For this review, take the finished solid that the model builds, in its own axes (mm). A direction names the side the tool comes from. Give positions to 0.01 mm unless a question says otherwise; leave off trailing zeros. Loops run counter-clockwise (first coordinate to the right, second up) from the corner with the lowest first, then second, coordinate; pieces in that order, holes last. Notation, with made-up numbers: M 11.5,60 L 16.5,60 A20 cw 16.5,99 Z; hole C 20.25,9 d2. An arc over 180 degrees is marked long. Use CSV: the item, a comma, the result in double quotes. Start each with the question number.
1. To check wall thickness, follow line 1 (X direction, y = -16, z = 1.65); line 2 (X direction, y = 78, z = -4); line 3 (Z direction, x = -7, y = -17). State the ranges of each line that lie inside material, in increasing order. Write a range as [from, to].
2. Take a section at A-A, the plane y = 31.5. Write out the cut boundary in (x, z), and give its area (3 significant figures).
3. Insertion check: P1, Ø12, axis at y = 23.5, z = -4.5, coming from the +X side; P2, Ø1.7, axis at x = 3.85, y = -22.66, coming from the -Z side; P3, Ø8, axis at x = -1, y = -6, coming from the +Z side. Each pin has a flat end and moves straight along its axis. Give the tip position at first contact, or say it passes through.
4. Take a section at B-B, the plane z = 25.5. Write out the cut boundary in (x, y), and give its area (3 significant figures).
5. Tool access review of faces 1 (the face through (-17, 66, 2)), 2 (the face through (-2, 0, 2)), 3 (the face through (-7, -5, 3)), 4 (the face through (-15, 50, -20)), 5 (the face through (-16, 100, 2)): name each direction out of +Z, -Z, +X, -X, +Y, -Y from which nothing blocks a thin tool from reaching the whole face with its end or side.
Autodesk Inventor part; units mm, degrees
ref_plane "YZ Plane" through (0, 0, 0) normal (1, 0, 0) x (0, 1, 0)
ref_plane "XZ Plane" through (0, 0, 0) normal (0, 1, 0) x (-1, 0, 0)
ref_plane "XY Plane" through (0, 0, 0) normal (0, 0, 1) x (1, 0, 0)
sketch "Sketch1" plane through (0, 0, 0) normal (0, 0, 1) x (1, 0, 0)
  line L0 (-9, 25) -> (9, 25)
  line L1 (9, 25) -> (9, -25)
  line L2 (9, -25) -> (-9, -25)
  line L3 (-9, -25) -> (-9, 25)
  point P0 (0, 0)
  point P1 (0, 25)
  point P2 (-9, 0)
  dimension "d0" = 18
  dimension "d1" = 50
extrude "Extrusion1" add sketch "Sketch1" along normal blind 3
sketch "Sketch2" plane through (0, 0, 3) normal (0, 0, 1) x (1, 0, 0)
  circle A0 centre (0, -16) radius 9
  circle A1 centre (0, 16) radius 9
  line L0 (-9, -25) -> (9, -25)
  circle A2 centre (0, -8.304) radius 0.75
  line L1 (9, 25) -> (-9, 25)
  point P0 (0, 0)
  point P1 (-4, -25)
  point P2 (4, -25)
  point P3 (4, 25)
  point P4 (-4, 25)
  dimension "d6" = 18
  dimension "d8" = 1.5
  dimension "d10" = 18
extrude "Extrusion2" cut sketch "Sketch2" against normal up to surface (3 mm away) contours A2
pattern_circular "Circular Pattern1" count 12 over 360 about axis through (0, -16, 3) along (0, 0, 1) of "Extrusion2"
sketch "Sketch7" plane through (0, 0, 3) normal (0, 0, 1) x (1, 0, 0)
  line L0 (-19, 0) -> (11, 0)
  line L1 (11, 0) -> (11, 28.3489)
  line L2 (11, 28.3489) -> (-19, 28.3489)
  line L3 (-19, 28.3489) -> (-19, 0)
  line L4 (-9, -25) -> (9, -25)
  line L5 (-9, 25) -> (-9, -25)
  line L6 (9, -25) -> (9, 25)
  point P0 (0, 0)
  point P1 (-4, -25)
  point P2 (4, -25)
  point P3 (-9, 20)
  point P4 (-9, -20)
  point P5 (9, -20)
  dimension "d44" = 25
  dimension "d48" = 30
  dimension "d49" = 2
extrude "Extrusion8" cut sketch "Sketch7" against normal up to surface (3 mm away) contours L3 L2 L1 L0
ref_plane "Work Plane1" through (-9, -20, 0) normal (-1, 0, 0) x (0, 0, 1)
sketch "Sketch9" plane through (-9, -20, 0) normal (-1, 0, 0) x (0, 0, 1)
  line L0 (3, 0) -> (3, 20)
  line L1 (3, 20) -> (0, 20)
  line L2 (0, 20) -> (0, 0)
  line L3 (3, 0) -> (3, -5)
  line L4 (3, -5) -> (0, -5)
  line L5 (0, -5) -> (3, -5)
  line L6 (0, -5) -> (0, 0)
extrude "Extrusion9" add sketch "Sketch9" along normal blind 8
fillet "Fillet3" radius 5 1 edges at (9, -25, 1.5)
sketch "Sketch10" plane through (9, 0, 3) normal (0, 1, 0) x (1, 0, 0)
  line L0 (-5, 3) -> (-26, 3)
  line L1 (-26, 0) -> (-23, 0)
  line L2 (-23, 0) -> (-23, 3)
  line L3 (-23, 3) -> (-26, 3)
  line L4 (-26, 3) -> (-26, 0)
  point P0 (-9, 3)
  dimension "d53" = 3
extrude "Extrusion10" add sketch "Sketch10" along normal blind 70
fillet "Fillet4" radius 5 1 edges at (-17, -25, 1.5)
sketch "Sketch11" plane through (0, 0, 3) normal (0, 0, 1) x (1, 0, 0)
  line L0 (-14, 0) -> (-14, 70)
  line L1 (-17, 70) -> (-14, 70)
  line L2 (-14, 70) -> (-14, 50)
  line L3 (-14, 50) -> (-17, 50)
  line L4 (-17, 50) -> (-17, 70)
  point P0 (0, 0)
  dimension "d57" = 20
extrude "Extrusion11" add sketch "Sketch11" along normal blind 30
sketch "Sketch12" plane through (0, 0, 0) normal (0, 0, -1) x (-1, 0, 0)
  line L0 (14, 0) -> (14, 70)
  line L1 (17, 70) -> (14, 70)
  line L2 (14, 70) -> (14, 50)
  line L3 (14, 50) -> (17, 50)
  line L4 (17, 50) -> (17, 70)
  point P0 (0, 0)
  dimension "d60" = 20
extrude "Extrusion12" add sketch "Sketch12" along normal blind 30
sketch "Sketch13" plane through (9, 70, 3) normal (0, 1, 0) x (1, 0, 0)
  line L0 (-26, 33) -> (-23, 33)
  line L1 (-23, 33) -> (-23, -30)
  line L2 (-23, -30) -> (-26, -30)
  line L3 (-26, -30) -> (-26, 33)
  point P0 (-9, 3)
extrude "Extrusion13" add sketch "Sketch13" along normal blind 30
sketch "Sketch14" plane through (0, 0, 33) normal (0, 0, 1) x (1, 0, 0)
  line L0 (-17, 50) -> (-14, 50)
  line L1 (-14, 50) -> (-14, 100)
  line L2 (-14, 100) -> (-17, 100)
  line L3 (-17, 100) -> (-17, 50)
  point P0 (0, 0)
extrude "Extrusion14" add sketch "Sketch14" along normal blind 10
sketch "Sketch15" plane through (0, 0, -30) normal (0, 0, -1) x (-1, 0, 0)
  line L0 (17, 100) -> (14, 100)
  line L1 (14, 100) -> (14, 50)
  line L2 (14, 50) -> (17, 50)
  line L3 (17, 50) -> (17, 100)
  point P0 (0, 0)
extrude "Extrusion15" add sketch "Sketch15" along normal blind 10
properties part number "second_perc_link"
Result set:
1,line 1,"[-17, -8.45], [-6.95, 6.95], [8.45, 9]"
1,line 2,"[-17, -14]"
1,line 3,"[0, 3]"
2,outline,"M -17,0 L -14,0 L -14,3 L -17,3 Z"
2,area,"9.00 mm2"
3,P1,"x = -14"
3,P2,"z = 0"
3,P3,"z = 3"
4,outline,"M -17,50 L -14,50 L -14,100 L -17,100 Z"
4,area,"150 mm2"
5,face 1,"+Z, -Z, -X, +Y, -Y"
5,face 2,"+Z, -Z, +X, +Y"
5,face 3,"+Z, +X, -X, -Y"
5,face 4,"-Z, +X, -X, -Y"
5,face 5,"+Z, -Z, +X, -X, +Y"
